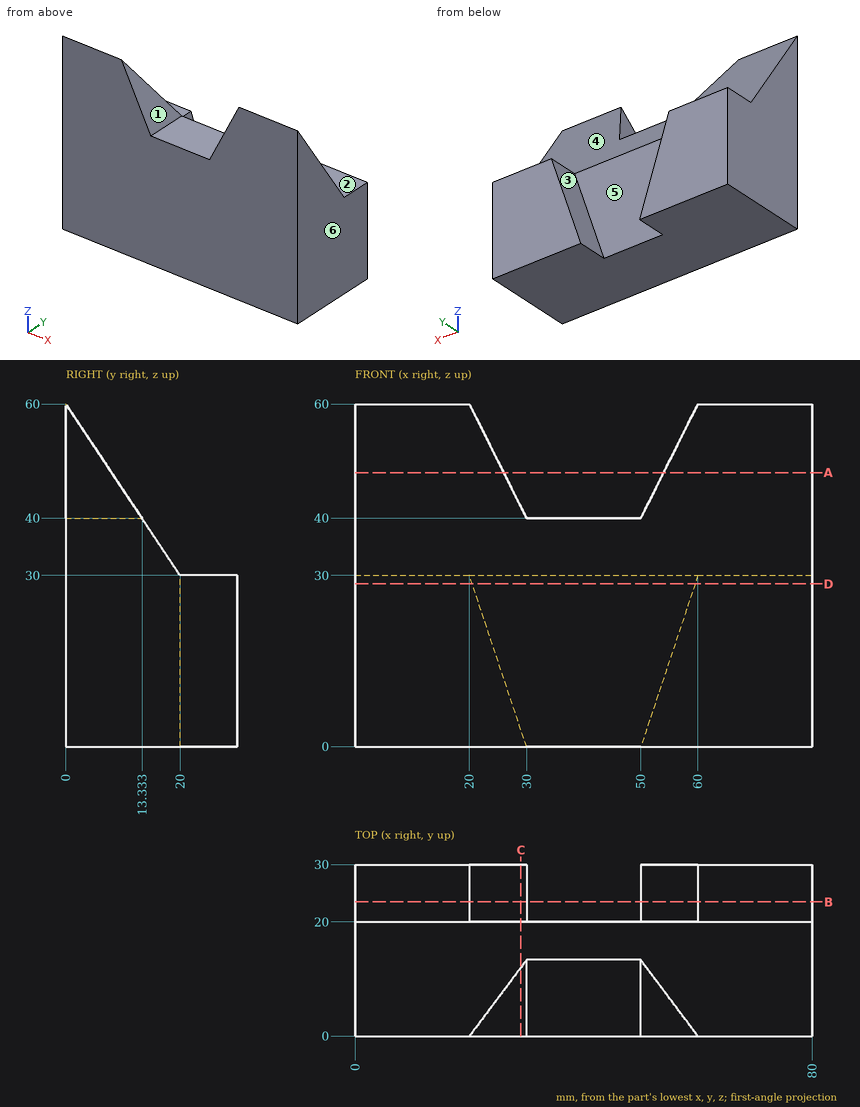
Geometry: see drawing. Coordinates: mm, zero at the bounding-box minimum. A direction names the side the tool comes from. Round coordinates to 2 decimals unless told otherwise and drop trailing zeros. Write each loop counter-clockwise with the first axis right and the second up, starting at its lowest first coordinate (ties: lowest second). Pieces come first, ordered by that corner, then holes. Notation, with made-up numbers: (-10.5, 15) -> (3.5, 15) arc R28 ccw to (3.5, 42) -> close; hole circle Ø3 at (64, 43). An arc over 180 degrees is marked (long way). Answer as CSV lines item,"result".
1. Section C-C (x = 29). Return the cut outline in (y, z), plus the area to 3 significant figures.
Geometry says:
outline,"(0, 0) -> (30, 0) -> (30, 3) -> (20, 3) -> (20, 30) -> (12, 42) -> (0, 42) -> close"
area,"822 mm^2"
2. Ray query, L1, parallel to Y at x = 43.5, z = 9; L2, parallel to X at y = 5.25, z = 48; L3, parallel to Z at x = 45, y = 6.75. Return the intervals inside material, ascending. Write a range as [from, to].
Geometry says:
L1,"y = [0, 20]"
L2,"x = [0, 26], [54, 80]"
L3,"z = [0, 40]"
3. Reachability of the marked faces 1, 2 and 3 from +Z, -Z, +X, -X, +Y, -Y: full face, straight path, thin tool, end or side. Return the list, or none.
Geometry says:
face 1,"+Z, +Y, -Y"
face 2,"+Z, +X, -X, +Y"
face 3,"+Z, +Y"
4. Section D-D (z = 28.5). Return the cut outline in (x, y), plus the area to 3 significant figures.
Geometry says:
outline,"(0, 0) -> (80, 0) -> (80, 30) -> (59.5, 30) -> (59.5, 20) -> (20.5, 20) -> (20.5, 30) -> (0, 30) -> close"
area,"2,010 mm^2"
5. Mould query, pull axis X, two halves, no side actions, for the marked faces 4, 5 and 6. Classes: +X half, -X half, draft (parallel to the pull), parting line (faces both ways), or undercut.
Geometry says:
face 4,"draft"
face 5,"undercut"
face 6,"+X half"
6. Contact query for flat-ended pins moving along their axis: P1, Ø2, axis at x = 67, z = 8, coming from the -Y side; P2, Ø9, axis at x = 43, z = 8.5, coming from the +Y side; P3, Ø8, axis at x = 67.5, y = 26, coming from the +Z side; P4, Ø6.5, axis at x = 40, y = 9, coming from the +Z side. Output: stop coordinate, or through.
Geometry says:
P1,"stops at y = 0"
P2,"stops at y = 20"
P3,"stops at z = 30"
P4,"stops at z = 40"
7. Section B-B (y = 23.5). Return the cut outline in (x, z).
Geometry says:
outline,"(0, 0) -> (30, 0) -> (20, 30) -> (0, 30) -> close; (50, 0) -> (80, 0) -> (80, 30) -> (60, 30) -> close"
8. Section A-A (z = 48). Return the cut outline in (x, y), plus the area to 3 significant figures.
Geometry says:
outline,"(0, 0) -> (26, 0) -> (26, 8) -> (0, 8) -> close; (54, 0) -> (80, 0) -> (80, 8) -> (54, 8) -> close"
area,"416 mm^2"
